```python
from build123d import *

# Parameters (mm, degrees)
SKETCH_1_W           = 230
SKETCH_1_H           = 79
EXTRUDE_1_DEPTH      = 3
EXTRUDE_2_DEPTH      = 3
EXTRUDE_2_DEPTH_BACK = 233
SKETCH_4_W           = 3
SKETCH_4_H           = 35
SKETCH_2_R           = 1.5
CUT_EXTRUDE_1_DEPTH  = 3
SKETCH_3_R           = 1.5
CUT_EXTRUDE_2_DEPTH  = 3
SKETCH_5_W           = 3
SKETCH_5_H           = 15
CUT_EXTRUDE_3_DEPTH  = 3
CUT_EXTRUDE_4_DEPTH  = 3
SKETCH_8_W           = 10
SKETCH_8_H           = 3
EXTRUDE_3_DEPTH      = 3
SKETCH_9_W           = 40
SKETCH_9_H           = 3
EXTRUDE_4_DEPTH      = 3
CUT_EXTRUDE_5_DEPTH  = 3
CUT_EXTRUDE_6_DEPTH  = 3
SKETCH_12_W          = 19
SKETCH_12_H          = 13
CUT_EXTRUDE_7_DEPTH  = 10


with BuildPart() as part:
    # Эскиз1 → Бобышка-Вытянуть1 (new body)
    with BuildSketch(Plane.XY):
        with Locations((115, 39.5)):
            Rectangle(SKETCH_1_W, SKETCH_1_H)
    extrude(amount=EXTRUDE_1_DEPTH)

    # Эскиз4 → Бобышка-Вытянуть2 (add, two sides: drawn at the far end of the back side and taken through both)
    with BuildSketch(Plane(origin=(230, 0, 0), x_dir=(0, 0, -1), z_dir=(1, 0, 0)).offset(-EXTRUDE_2_DEPTH_BACK)):
        with Locations((-1.5, 35)):
            Rectangle(SKETCH_4_W, SKETCH_4_H)
    extrude(amount=EXTRUDE_2_DEPTH + EXTRUDE_2_DEPTH_BACK)

    # Эскиз2 → Вырез-Вытянуть1 (cut)
    with BuildSketch(Plane.XY.offset(3)):
        with Locations((65, 35)):
            Circle(SKETCH_2_R)
        with Locations((165, 35)):
            Circle(SKETCH_2_R)
    extrude(amount=-CUT_EXTRUDE_1_DEPTH, mode=Mode.SUBTRACT)

    # Эскиз3 → Вырез-Вытянуть2 (cut)
    with BuildSketch(Plane.XY.offset(3)):
        with Locations((33.5, 52.5)):
            Circle(SKETCH_3_R)
        with Locations((196.5, 52.5)):
            Circle(SKETCH_3_R)
        with Locations((196.5, 17.5)):
            Circle(SKETCH_3_R)
        with Locations((33.5, 17.5)):
            Circle(SKETCH_3_R)
    extrude(amount=-CUT_EXTRUDE_2_DEPTH, mode=Mode.SUBTRACT)

    # Эскиз5 → Вырез-Вытянуть3 (cut)
    with BuildSketch(Plane.XY.offset(3)):
        with Locations((33.5, 35)):
            Rectangle(SKETCH_5_W, SKETCH_5_H)
        with Locations((196.5, 35)):
            Rectangle(SKETCH_5_W, SKETCH_5_H)
    extrude(amount=-CUT_EXTRUDE_3_DEPTH, mode=Mode.SUBTRACT)

    # Эскиз6 → Вырез-Вытянуть4 (cut)
    with BuildSketch(Plane.XY.offset(3)):
        Polygon((0, 10.25), (6, 10.25), (6, 11.5), (8.5, 11.5), (8.5, 10.25), (14.5, 10.25), (14.5, 7.25), (8.5, 7.25), (8.5, 6), (6, 6), (6, 7.25), (0, 7.25), align=None)
        Polygon((230, 7.25), (230, 10.25), (224, 10.25), (224, 11.5), (221.5, 11.5), (221.5, 10.25), (215.5, 10.25), (215.5, 7.25), (221.5, 7.25), (221.5, 6), (224, 6), (224, 7.25), align=None)
        Polygon((230, 59.75), (224, 59.75), (224, 58.5), (221.5, 58.5), (221.5, 59.75), (215.5, 59.75), (215.5, 62.75), (221.5, 62.75), (221.5, 64), (224, 64), (224, 62.75), (230, 62.75), align=None)
        Polygon((0, 62.75), (0, 59.75), (6, 59.75), (6, 58.5), (8.5, 58.5), (8.5, 59.75), (14.5, 59.75), (14.5, 62.75), (8.5, 62.75), (8.5, 64), (6, 64), (6, 62.75), align=None)
    extrude(amount=-CUT_EXTRUDE_4_DEPTH, mode=Mode.SUBTRACT)

    # Эскиз8 → Бобышка-Вытянуть3 (add)
    with BuildSketch(Plane(origin=(0, 79, 0), x_dir=(1, 0, 0), z_dir=(0, 1, 0))):
        with Locations((221, -1.5)):
            Rectangle(SKETCH_8_W, SKETCH_8_H)
        with Locations((9, -1.5)):
            Rectangle(SKETCH_8_W, SKETCH_8_H)
    extrude(amount=EXTRUDE_3_DEPTH)

    # Эскиз9 → Бобышка-Вытянуть4 (add)
    with BuildSketch(Plane(origin=(0, 79, 0), x_dir=(1, 0, 0), z_dir=(0, 1, 0))):
        with Locations((115, -1.5)):
            Rectangle(SKETCH_9_W, SKETCH_9_H)
    extrude(amount=EXTRUDE_4_DEPTH)

    # Эскиз10 → Вырез-Вытянуть5 (cut)
    with BuildSketch(Plane.XY.offset(3)):
        Polygon((55.5, 79), (55.5, 73), (54.25, 73), (54.25, 70.5), (55.5, 70.5), (55.5, 64.5), (58.5, 64.5), (58.5, 70.5), (59.75, 70.5), (59.75, 73), (58.5, 73), (58.5, 79), align=None)
        Polygon((171.5, 79), (174.5, 79), (174.5, 73), (175.75, 73), (175.75, 70.5), (174.5, 70.5), (174.5, 64.5), (171.5, 64.5), (171.5, 70.5), (170.25, 70.5), (170.25, 73), (171.5, 73), align=None)
    extrude(amount=-CUT_EXTRUDE_5_DEPTH, mode=Mode.SUBTRACT)

    # Эскиз11 → Вырез-Вытянуть6 (cut)
    with BuildSketch(Plane.XY.offset(3)):
        with BuildLine():
            Line((78.5, 56.5), (151.5, 56.5))
            ThreePointArc((151.5, 56.5), (152.914213562, 55.914213562), (153.5, 54.5))
            Line((153.5, 54.5), (153.5, 15.5))
            ThreePointArc((153.5, 15.5), (152.914213562, 14.085786438), (151.5, 13.5))
            Line((151.5, 13.5), (78.5, 13.5))
            ThreePointArc((78.5, 13.5), (77.085786438, 14.085786438), (76.5, 15.5))
            Line((76.5, 15.5), (76.5, 54.5))
            ThreePointArc((76.5, 54.5), (77.085786438, 55.914213562), (78.5, 56.5))
        make_face()
    extrude(amount=-CUT_EXTRUDE_6_DEPTH, mode=Mode.SUBTRACT)

    # Эскиз12 → Вырез-Вытянуть7 (cut)
    with BuildSketch(Plane(origin=(0, 0, 0), x_dir=(-1, 0, 0), z_dir=(0, 0, -1))):
        with Locations((-115, 67)):
            Rectangle(SKETCH_12_W, SKETCH_12_H)
    extrude(amount=-CUT_EXTRUDE_7_DEPTH, mode=Mode.SUBTRACT)


solid = part.part
```
Geometry check sheet. Reference: the model listing, model coordinates, mm. Round coordinates to 2 decimals unless told otherwise and drop trailing zeros. Loops run counter-clockwise (first coordinate to the right, second up) from the corner with the lowest first, then second, coordinate; pieces in that order, holes last. Notation, with made-up numbers: (31.25, 67) - (73.25, 67) arc R23 ccw to (73.25, 75) - close; hole circle Ø2 at (5.25, 37.5). An arc over 180 degrees is marked (long way). Write item = value, one per line. Start each with the question number.
1. Section check A-A on y = 30. Enter the section's corners in (x, z), then the cut area to 3 significant figures.
2. Section check B-B on x = 140. Enter the section's corners in (y, z), then the cut area to 3 significant figures.
3. Thickness scan on line 1 (X direction, y = 72, z = 2.85); line 2 (Y direction, x = 33.5, z = 2.15); line 3 (X direction, y = 66.5, z = 1.85). Record the ranges inside material, lowest first.
4. Section check C-C on x = 115. Enter the section's corners in (y, z).
5. Depth check by flat-ended pin: pin 1 (0.6 mm diameter, centred on y = 59, z = 2, fed in from +X); pin 2 (1 mm diameter, centred on x = 175, z = 1.5, fed in from +Y); pin 3 (0.6 mm diameter, centred on y = 63.5, z = 1, fed in from -X). Enter the tip coordinate at first touch or a pass-through.
6. Section check D-D on z = 0.65. Give the number of separate pieces and of enclosed holes in the cut face, then the cut area to 3 significant figures.
Working result:
q1.outline = (-3, 0) - (32, 0) - (32, 3) - (-3, 3) - close; (35, 0) - (76.5, 0) - (76.5, 3) - (35, 3) - close; (153.5, 0) - (195, 0) - (195, 3) - (153.5, 3) - close; (198, 0) - (233, 0) - (233, 3) - (198, 3) - close
q1.area = 459 mm^2
q2.outline = (0, 0) - (13.5, 0) - (13.5, 3) - (0, 3) - close; (56.5, 0) - (79, 0) - (79, 3) - (56.5, 3) - close
q2.area = 108 mm^2
q3.line_1 = 0 to 54.25, 59.75 to 105.5, 124.5 to 170.25, 175.75 to 230
q3.line_2 = 0 to 16, 19 to 27.5, 42.5 to 51, 54 to 79
q3.line_3 = 0 to 55.5, 58.5 to 105.5, 124.5 to 171.5, 174.5 to 230
q4.outline = (0, 0) - (13.5, 0) - (13.5, 3) - (0, 3) - close; (56.5, 0) - (60.5, 0) - (60.5, 3) - (56.5, 3) - close; (73.5, 0) - (82, 0) - (82, 3) - (73.5, 3) - close
q5.pin_1 = 230
q5.pin_2 = 79
q5.pin_3 = 0
q6.separate_pieces = 1
q6.enclosed_holes = 10
q6.area = 14,600 mm^2
